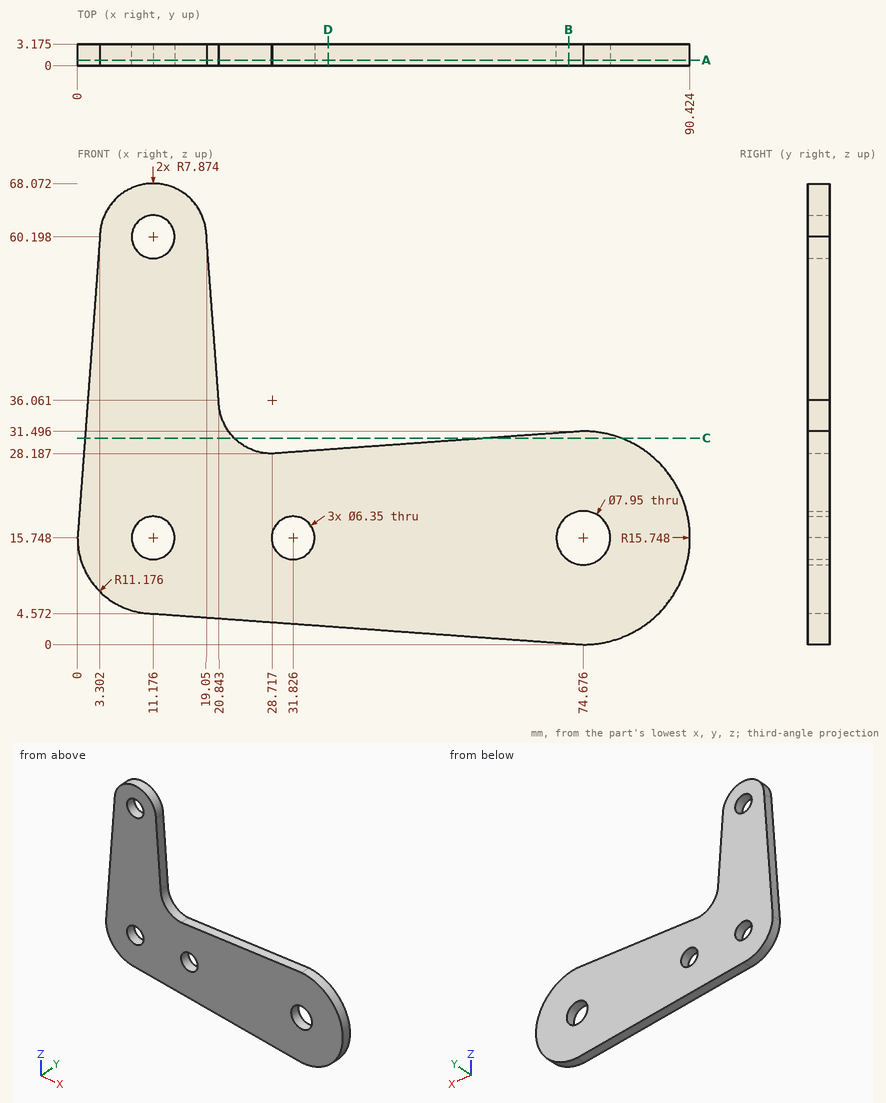
Verification items for this drawing (mm, ordinates from the low corner). Give positions to 0.01 mm unless a question says otherwise; leave off trailing zeros. Order: outer loops, then holes, each group sorted by start corner. A loop starts at its lowest first (then second) coordinate and runs counter-clockwise, first axis right, second up. Notation, with made-up numbers: M -10,-30 L 18,-30 A17 cw 18,-23 Z; hole C 66,80.5 d1. An arc over 180 degrees is marked long. Use a Markdown table: item, result.
Item 1: Section check B-B (x = 72.5). Record the cut outline in (y, z) (1 decimal), and give its area (3 significant figures).
Answers follow:
| item | result |
|---|---|
| outline | M 0,0.2 L 3.2,0.2 L 3.2,12.4 L 0,12.4 Z; M 0,19.1 L 3.2,19.1 L 3.2,31.3 L 0,31.3 Z |
| area | 77.9 mm2 |
Item 2: Material ranges on line 1 along X through (y, z) = (1.15, 17.5) (1 decimal); line 2 along Z through (x, y) = (9.5, 3.05) (1 decimal); line 3 along Z through (x, y) = (32.5, 0.25) (1 decimal), recorded low to high.
Answers follow:
| item | result |
|---|---|
| line 1 | x = 0.1 to 8.5, 13.8 to 29.2, 34.5 to 71.1, 78.2 to 90.3 |
| line 2 | z = 4.7 to 13.1, 18.4 to 57.5, 62.9 to 67.9 |
| line 3 | z = 3 to 12.6, 18.9 to 28.5 |
Item 3: Section check C-C (z = 30.5). Record the cut outline in (x, y) (1 decimal).
Answers follow:
| item | result |
|---|---|
| outline | M 1.1,0 L 23.1,0 L 23.1,3.2 L 1.1,3.2 Z; M 60.8,0 L 80.2,0 L 80.2,3.2 L 60.8,3.2 Z |
Item 4: Section check D-D (x = 37). Record the cut outline in (y, z) (1 decimal).
Answers follow:
| item | result |
|---|---|
| outline | M 0,2.7 L 3.2,2.7 L 3.2,28.8 L 0,28.8 Z |
Item 5: Depth check by flat-ended pin: P1, Ø1, axis at y = 1, z = 51.5, coming from the +X side; P2, Ø5.5, axis at x = 31.83, z = 15.75, coming from the +Y side. Enter the tip coordinate at first touch or a pass-through.
Answers follow:
| item | result |
|---|---|
| P1 | stops at x = 19.73 |
| P2 | passes through |
Item 6: Section check A-A (y = 0.8). State how many separate pieces and enclosed holes the cut face has, and give its area (3 significant figures).
Answers follow:
| item | result |
|---|---|
| separate pieces | 1 |
| enclosed holes | 4 |
| area | 2,890 mm2 |
